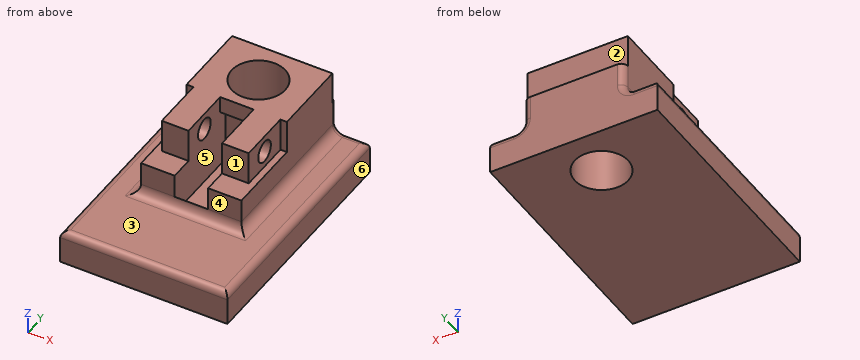
```python
from build123d import *

# Parameters (mm, degrees)
SKETCH1_W           = 125
SKETCH1_H           = 180
BASE_EXTRUDE_DEPTH  = 25
SKETCH2_W           = 75
SKETCH2_H           = 120
BOSS_EXTRUDE1_DEPTH = 25
FILLET2_R           = 7.5
FILLET4_R           = 5
SKETCH4_W           = 75
SKETCH4_H           = 57.5
BOSS_EXTRUDE2_DEPTH = 25
SKETCH7_R           = 20
CUT_EXTRUDE2_DEPTH  = 105
SKETCH8_W           = 20
SKETCH8_H           = 40
BOSS_EXTRUDE4_DEPTH = 25
SKETCH9_R           = 8
CUT_EXTRUDE3_DEPTH  = 89
SKETCH10_W          = 25
SKETCH10_H          = 57.5
CUT_EXTRUDE4_DEPTH  = 31
SKETCH12_W          = 25
SKETCH12_H          = 43.423813554
CUT_EXTRUDE6_DEPTH  = 7


with BuildPart() as part:
    # Sketch1 → Base-Extrude (new body)
    with BuildSketch(Plane.XY):
        with Locations((-7.794747082, 12.712840467)):
            Rectangle(SKETCH1_W, SKETCH1_H)
    extrude(amount=BASE_EXTRUDE_DEPTH)

    # Sketch2 → Boss-Extrude1 (add)
    with BuildSketch(Plane.XY.offset(25)):
        with Locations((-7.794747082, 42.712840467)):
            Rectangle(SKETCH2_W, SKETCH2_H)
    extrude(amount=BOSS_EXTRUDE1_DEPTH)

    # Fillet2
    fillet2_edges = [part.edges().sort_by_distance(p)[0] for p in [
        (-45.294747082, 42.712840467, 25),
        (-7.794747082, -17.287159533, 25),
        (29.705252918, 42.712840467, 25),
    ]]
    fillet(fillet2_edges, radius=FILLET2_R)

    # Fillet4
    fillet4_edges = [part.edges().sort_by_distance(p)[0] for p in [
        (54.705252918, 12.712840467, 25),
        (-61.544747082, 102.712840467, 25),
        (-45.294747082, 102.712840467, 41.25),
        (29.705252918, 102.712840467, 41.25),
        (31.901952059, 102.712840467, 27.196699141),
        (-47.491446223, 102.712840467, 27.196699141),
        (-70.294747082, 12.712840467, 25),
        (-7.794747082, -77.287159533, 25),
    ]]
    fillet(fillet4_edges, radius=FILLET4_R)

    # Sketch4 → Boss-Extrude2 (add)
    with BuildSketch(Plane.XY.offset(50)):
        with Locations((-7.794747082, 68.962840467)):
            Rectangle(SKETCH4_W, SKETCH4_H)
    extrude(amount=BOSS_EXTRUDE2_DEPTH)

    # Sketch7 → Cut-Extrude2 (cut)
    with BuildSketch(Plane.XY.offset(75)):
        with Locations((-7.794747082, 67.712840467)):
            Circle(SKETCH7_R)
    extrude(amount=-CUT_EXTRUDE2_DEPTH, mode=Mode.SUBTRACT)

    # Sketch8 → Boss-Extrude4 (add)
    with BuildSketch(Plane.XY.offset(50)):
        with Locations((-30.180989309, 20.212840467)):
            Rectangle(SKETCH8_W, SKETCH8_H)
        with Locations((14.819010691, 20.212840467)):
            Rectangle(SKETCH8_W, SKETCH8_H)
    extrude(amount=BOSS_EXTRUDE4_DEPTH)

    # Sketch9 → Cut-Extrude3 (cut)
    with BuildSketch(Plane(origin=(24.819010691, 0, 0), x_dir=(0, 0, -1), z_dir=(1, 0, 0))):
        with Locations(Location((-62.5, 20.212840467, 0), (0, 0, 90))):
            Circle(SKETCH9_R)
    extrude(amount=-CUT_EXTRUDE3_DEPTH, mode=Mode.SUBTRACT)

    # Sketch10 → Cut-Extrude4 (cut)
    with BuildSketch(Plane.XY.offset(50)):
        with Locations((-7.680989309, 11.462840467)):
            Rectangle(SKETCH10_W, SKETCH10_H)
    extrude(amount=-CUT_EXTRUDE4_DEPTH, mode=Mode.SUBTRACT)

    # Sketch12 → Cut-Extrude6 (cut)
    with BuildSketch(Plane.XZ.offset(-40.212840467)):
        with Locations((-7.680989309, 40.711906777)):
            Rectangle(SKETCH12_W, SKETCH12_H)
    extrude(amount=-CUT_EXTRUDE6_DEPTH, mode=Mode.SUBTRACT)


solid = part.part
```
The model under review builds one solid part; all positions refer to its coordinate system, in mm. Face numbers are marked on the shaded views. A direction names the side the tool comes from. Round coordinates to 2 decimals unless told otherwise and drop trailing zeros. Write each loop counter-clockwise with the first axis right and the second up, starting at its lowest first coordinate (ties: lowest second). Pieces come first, ordered by that corner, then holes. Notation, with made-up numbers: M 39.25,-31.75 L 87.25,-31.75 A11 cw 87.25,-10.75 Z; hole C 63,-17.75 d4. An arc over 180 degrees is marked long. Use CSV: the item, a comma, the result in double quotes. Start each with the question number.
(1) The part is to be moulded in two halves that separate along Y. For the marked faces 4, 5 and 6, say which applies: +Y half, -Y half, draft (parallel to the pull), parting line (faces both ways), or undercut.
(2) We need section D-D, the plane y = -63.5. State the section outline as (x, z) points.
(3) We need section C-C, the plane y = 78. State the section outline as (x, z) points, then the cut area to 3 significant figures.
(4) We need section B-B, the plane x = 46.5. State the section outline as (y, z) points.
(5) Clearance check with flat-ended pins moving along their axes: P1, Ø7.5, axis at y = 30, z = 60, coming from the -X side; P2, Ø20, axis at y = 14.5, z = 65, coming from the +X side; P3, Ø2.5, axis at x = -43, z = 58.5, coming from the -Y side. State where each tip first meets the part, or that it passes through.
(6) Tool access review of the marked faces 1, 2 and 3: name each direction out of +Z, -Z, +X, -X, +Y, -Y from which nothing blocks a thin tool from reaching the whole face with its end or side.
(7) We need section A-A, the plane y = 38. State the section outline as (x, z) points.
(8) For line 1 along X through (y, z) = (32.5, 69.5); line 2 along Z through (x, y) = (6.5, -35); line 3 along X through (y, z) = (93.5, 39.5), list the stretches that pass through material, from the lowest coordinate up.
Findings:
1,face 4,"-Y half"
1,face 5,"undercut"
1,face 6,"draft"
2,outline,"M -70.29,0 L 54.71,0 L 54.71,20 A5 ccw 49.71,25 L -65.29,25 A5 ccw -70.29,20 Z"
3,outline,"M -70.29,0 L -24.95,0 L -24.95,75 L -45.29,75 L -45.29,32.5 A7.5 cw -52.79,25 L -65.29,25 A5 ccw -70.29,20 Z; M 9.36,0 L 54.71,0 L 54.71,20 A5 ccw 49.71,25 L 37.21,25 A7.5 cw 29.71,32.5 L 29.71,75 L 9.36,75 Z"
3,area,"4,320 mm^2"
4,outline,"M -77.29,0 L 102.71,0 L 102.71,20 A5 ccw 97.71,25 L -72.29,25 A5 ccw -77.29,20 Z"
5,P1,"x = -40.18"
5,P2,"x = 24.82"
5,P3,"y = 40.21"
6,face 1,"+Z, +X, -X, -Y"
6,face 2,"+Z, +X, -X, +Y"
6,face 3,"+Z, -Y"
7,outline,"M -70.29,0 L 54.71,0 L 54.71,20 A5 ccw 49.71,25 L 37.21,25 A7.5 cw 29.71,32.5 L 29.71,50 L 24.82,50 L 24.82,75 L 4.82,75 L 4.82,19 L -20.18,19 L -20.18,75 L -40.18,75 L -40.18,50 L -45.29,50 L -45.29,32.5 A7.5 cw -52.79,25 L -65.29,25 A5 ccw -70.29,20 Z"
8,line 1,"-40.18 to -20.18, 4.82 to 24.82"
8,line 2,"0 to 25"
8,line 3,"-45.29 to 29.71"
